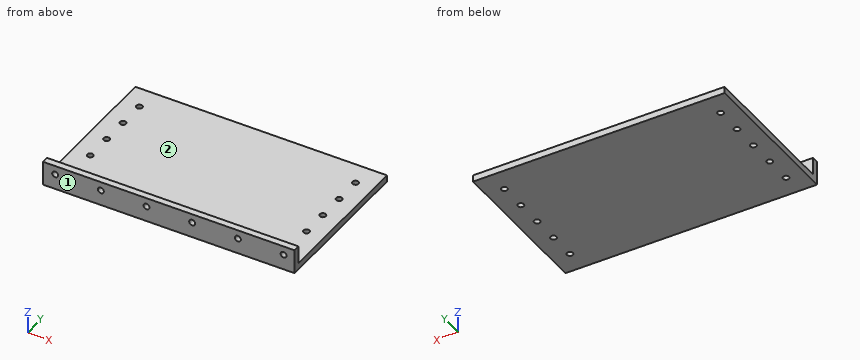
```python
from build123d import *

# Parameters (mm, degrees)
SKETCH1_W                       = 568
SKETCH1_H                       = 350
BOSS_EXTRUDE1_DEPTH             = 15
SKETCH4_W                       = 568
SKETCH4_H                       = 15
BOSS_EXTRUDE3_DEPTH             = 40
M12_CLEARANCE_HOLE2_D           = 13.5
M12_CLEARANCE_HOLE2_CSINK_D     = 13.55
M12_CLEARANCE_HOLE2_CSINK_ANGLE = 100
LPATTERN1_COUNT                 = 5
LPATTERN1_PITCH                 = 62
M12_CLEARANCE_HOLE3_D           = 13.5
M12_CLEARANCE_HOLE3_CSINK_D     = 13.55
M12_CLEARANCE_HOLE3_CSINK_ANGLE = 100
LPATTERN2_COUNT                 = 5
LPATTERN2_PITCH                 = 62
M12_CLEARANCE_HOLE4_D           = 13.5
M12_CLEARANCE_HOLE4_CSINK_D     = 13.55
M12_CLEARANCE_HOLE4_CSINK_ANGLE = 100
LPATTERN3_COUNT                 = 6
LPATTERN3_PITCH                 = 103.1


with BuildPart() as part:
    # Sketch1 → Boss-Extrude1 (new body)
    with BuildSketch(Plane.XY):
        Rectangle(SKETCH1_W, SKETCH1_H)
    extrude(amount=BOSS_EXTRUDE1_DEPTH)

    # Sketch4 → Boss-Extrude3 (add)
    with BuildSketch(Plane.XY.offset(15)):
        with Locations((0, -167.5)):
            Rectangle(SKETCH4_W, SKETCH4_H)
    extrude(amount=BOSS_EXTRUDE3_DEPTH)

    # M12 Clearance Hole2 (through all)
    with Locations(Plane.XY.offset(15)):
        with Locations((244, 123)):
            m12_clearance_hole2 = CounterSinkHole(M12_CLEARANCE_HOLE2_D / 2, M12_CLEARANCE_HOLE2_CSINK_D / 2, counter_sink_angle=M12_CLEARANCE_HOLE2_CSINK_ANGLE)

    # LPattern1: M12 Clearance Hole2 ×5
    with Locations(*[(0, -i * LPATTERN1_PITCH, 0) for i in range(1, LPATTERN1_COUNT)]):
        add(m12_clearance_hole2, mode=Mode.SUBTRACT)

    # M12 Clearance Hole3 (through all)
    with Locations(Plane(origin=(0, 0, 0), x_dir=(1, 0, 0), z_dir=(0, 0, -1))):
        with Locations((-244, -123)):
            m12_clearance_hole3 = CounterSinkHole(M12_CLEARANCE_HOLE3_D / 2, M12_CLEARANCE_HOLE3_CSINK_D / 2, counter_sink_angle=M12_CLEARANCE_HOLE3_CSINK_ANGLE)

    # LPattern2: M12 Clearance Hole3 ×5
    with Locations(*[(0, -i * LPATTERN2_PITCH, 0) for i in range(1, LPATTERN2_COUNT)]):
        add(m12_clearance_hole3, mode=Mode.SUBTRACT)

    # M12 Clearance Hole4 (through all)
    with Locations(Plane(origin=(0, -160, 0), x_dir=(1, 0, 0), z_dir=(0, 1, 0))):
        with Locations((259, -35)):
            m12_clearance_hole4 = CounterSinkHole(M12_CLEARANCE_HOLE4_D / 2, M12_CLEARANCE_HOLE4_CSINK_D / 2, counter_sink_angle=M12_CLEARANCE_HOLE4_CSINK_ANGLE)

    # LPattern3: M12 Clearance Hole4 ×6
    with Locations(*[(-i * LPATTERN3_PITCH, 0, 0) for i in range(1, LPATTERN3_COUNT)]):
        add(m12_clearance_hole4, mode=Mode.SUBTRACT)


solid = part.part
```
Source: CAD feature listing. Evaluate the final solid. Frame: model axes, mm. Face numbers are marked on the shaded views. A direction names the side the tool comes from. Round coordinates to 2 decimals unless told otherwise and drop trailing zeros. Write each loop counter-clockwise with the first axis right and the second up, starting at its lowest first coordinate (ties: lowest second). Pieces come first, ordered by that corner, then holes. Notation, with made-up numbers: M 7,-22 L 47,-22 A16 ccw 47,-14 Z; hole C 71.25,55.5 d7. An arc over 180 degrees is marked long. Answer as a JSON object with one key per item and string values. Group by question number.
(1) Section query B-B on x = -50.3. Output: boundary loops of the cut face in (y, z) (3 decimals), then the cut area to 3 significant figures.
(2) Section query C-C on z = 35. State how many separate pieces and enclosed holes the cut face has, then the cut area to 4 significant figures.
(3) Reachability of the marked faces 1 and 2 from +Z, -Z, +X, -X, +Y, -Y: full face, straight path, thin tool, end or side. Return the list, or none.
(4) Ray query, line 1 (Y direction, x = -244, z = 11.5); line 2 (X direction, y = -63, z = 4.75); line 3 (Z direction, x = -153.4, y = -166.5). Return the intervals inside material, ascending. Write a range as [from, to].
(5) Section query A-A on y = -1. Output: boundary loops of the cut face in (x, z) (3 decimals).
(6) Section query D-D on x = -118. Output: boundary loops of the cut face in (y, z).
(7) First-contact query: pin 1 (15.5 mm diameter, centred on x = -153.4, z = 35, fed in from +Y); pin 2 (11 mm diameter, centred on x = 244, y = 123, fed in from -Z); pin 3 (21.5 mm diameter, centred on x = 244, y = -1, fed in from +Z). Flat tips, straight axial feed; report the tip coordinate or a pass-through.
Computed values:
{
 "1": {"outline": "M -175,0 L 175,0 L 175,15 L -160,15 L -160,28.225 L -160.021,28.25 L -175,28.25 Z; M -175,41.75 L -160.021,41.75 L -160,41.775 L -160,55 L -175,55 Z", "area": "5,650 mm^2"},
 "2": {"separate pieces": "7", "enclosed holes": "0", "area": "7,305 mm^2"},
 "3": {"face 1": "+Z, -Z, +X, -X, -Y", "face 2": "+Z, +X, -X, +Y"},
 "4": {"line 1": "[-175, -131.75], [-118.25, -69.75], [-56.25, -7.75], [5.75, 54.25], [67.75, 116.25], [129.75, 175]", "line 2": "[-284, -250.75], [-237.25, 237.25], [250.75, 284]", "line 3": "[0, 28.25], [41.75, 55]"},
 "5": {"outline": "M -284,0 L -250.775,0 L -250.75,0.021 L -250.75,15 L -284,15 Z; M -237.25,0.021 L -237.225,0 L 237.25,0 L 237.25,14.979 L 237.225,15 L -237.25,15 Z; M 250.75,0 L 284,0 L 284,15 L 250.775,15 L 250.75,14.979 Z"},
 "6": {"outline": "M -175,0 L 175,0 L 175,15 L -160,15 L -160,55 L -175,55 Z"},
 "7": {"pin 1": "y = -160", "pin 2": "through", "pin 3": "z = 15"}
}
